Verification items for this drawing (mm, ordinates from the low corner). Round coordinates to 2 decimals unless told otherwise and drop trailing zeros. One line per question, with ' | ' between items.
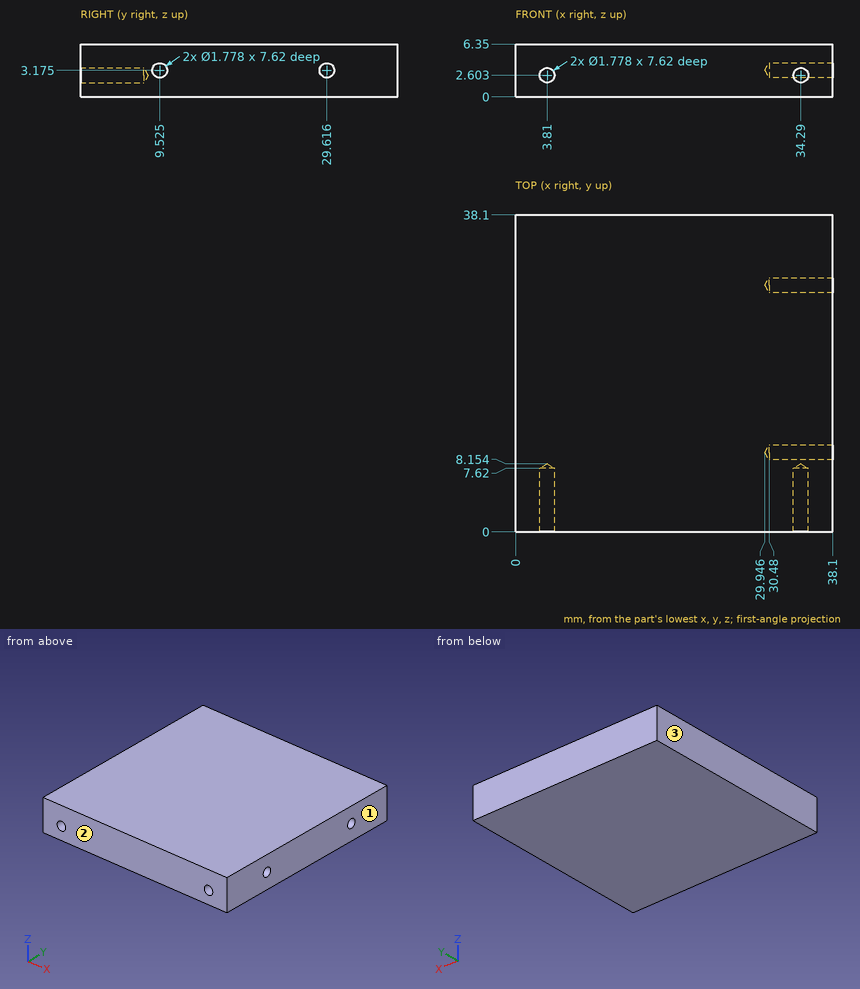
(1) Material ranges on line 1 (X direction, y = 2, z = 2.25) (1 decimal); line 2 (X direction, y = 10, z = 3.5); line 3 (Y direction, x = 4, z = 2.5) (1 decimal), recorded low to high.
Resolved:
line 1: x = 0 to 3, 4.6 to 33.5, 35.1 to 38.1 | line 2: x = 0 to 30.29 | line 3: y = 8 to 38.1
(2) Draft check along X on the marked faces 1, 2 and 3. Enter one of: +X half, -X half, draft (parallel to the pull), parting line (faces both ways), or undercut.
Resolved:
face 1: +X half | face 2: draft | face 3: -X half
(3) Go/stop test with flat-tipped pins: pin 1 (6 mm diameter, centred on x = 34, y = 24.5, fed in from -Z); pin 2 (1.4 mm diameter, centred on x = 3.81, z = 2.6, fed in from -Y). Record where each tip stops, or that it passes through.
Resolved:
pin 1: stops at z = 0 | pin 2: stops at y = 7.73
